Check sheet for the modelled part. Datum: model origin and axes. Units: mm. A direction names the side the tool comes from. Give positions to 0.01 mm unless a question says otherwise; leave off trailing zeros. Write each loop counter-clockwise with the first axis right and the second up, starting at its lowest first coordinate (ties: lowest second). Pieces come first, ordered by that corner, then holes. Notation, with made-up numbers: M -9,71.25 L -1,71.25 A32 ccw -1,103.25 Z; hole C 60,1 d2. An arc over 180 degrees is marked long. Write item = value, one per line. Start each with the question number.
1) Scan lines: L1, parallel to X at y = 25, z = 2; L2, parallel to X at y = 78.5, z = 4; L3, parallel to Y at x = -40, z = -15 (3 decimals). Record each from-to range of solid material in increasing order.
2) Sectioned sample at C-C, the plane y = 97. Record the cut outline in (x, z).
3) Gauge pin test, flat ends, axial feed: pin 1 (11 mm diameter, centred on x = 0, z = -22.225, fed in from +Y) (3 decimals); pin 2 (6 mm diameter, centred on x = -20.5, y = 72, fed in from -Z); pin 3 (5.5 mm diameter, centred on x = 31.81, z = 0, fed in from +Y). Record the tip position at first contact, or that the pin passes through.
4) Sectioned sample at B-B, the plane y = 25.4. Record the cut outline in (x, z).
5) Sectioned sample at A-A, the plane x = -31.75. Count the separate pieces of the cut face and the enclosed holes in it, then the cut area to 3 significant figures.
6) Draft check along X on faces 4 (the face through (10.554, 119.867, 1.612)), 5 (the face through (-1, 3.175, -16)), 6 (the face through (-44.45, 56, -3)). Enter one of: pulls with the +X half, pulls with the -X half, needs draft (parallel to the pull), parting line crosses it, or undercut.
7) Set-up check for faces 1 (the face through (44.45, 56, -3)), 2 (the face through (0.6, 119.062, 0.1)), 3 (the face through (21.4, 119.87, 3.23)): record each of +Z, -Z, +X, -X, +Y, -Y from which the full face is reachable in a straight line by a thin tool's end or side.
from build123d import *

# Parameters (mm, degrees)
SKETCH1_W               = 88.9
SKETCH1_H               = 12.7
BOSS_EXTRUDE1_DEPTH     = 76.2
SKETCH2_R               = 3.4925
BOSS_EXTRUDE4_DEPTH     = 3.175
BOSS_EXTRUDE5_DEPTH     = 12.7
CUT_EXTRUDE1_REACH      = 134.44
SKETCH4_R               = 3.4925
CUT_EXTRUDE2_DEPTH      = 133.439750453
CUT_EXTRUDE2_DEPTH_BACK = 133.439750453
SKETCH5_R               = 3.4925


with BuildPart() as part:
    # Sketch1 → Boss-Extrude1 (new body)
    with BuildSketch(Plane(origin=(0, 0, 0), x_dir=(1, 0, 0), z_dir=(0, 1, 0))):
        Rectangle(SKETCH1_W, SKETCH1_H)
    extrude(amount=BOSS_EXTRUDE1_DEPTH)

    # Sketch2 → Boss-Extrude4 (add)
    with BuildSketch(Plane(origin=(0, 0, 0), x_dir=(1, 0, 0), z_dir=(0, 1, 0))):
        Polygon((-44.45, 22.225), (-44.45, 6.35), (44.45, 6.35), (44.45, 31.75), (-44.45, 31.75), align=None)
        with Locations(Location((-25.4, 22.225, 0), (0, 0, 270))):
            Circle(SKETCH2_R, mode=Mode.SUBTRACT)
        with Locations(Location((0, 22.225, 0), (0, 0, 270))):
            Circle(SKETCH2_R, mode=Mode.SUBTRACT)
        with Locations(Location((25.4, 22.225, 0), (0, 0, 270))):
            Circle(SKETCH2_R, mode=Mode.SUBTRACT)
    extrude(amount=BOSS_EXTRUDE4_DEPTH)

    # Sketch3 → Boss-Extrude5 (add)
    with BuildSketch(Plane.XY.offset(6.35)):
        Polygon((-44.45, 76.2), (-44.45, 120.65), (44.45, 120.65), (44.45, 76.2), (42.8625, 76.2), (42.8625, 119.0625), (-42.8625, 119.0625), (-42.8625, 76.2), align=None)
    extrude(amount=-BOSS_EXTRUDE5_DEPTH)

    # Sketch4 → Cut-Extrude1 (cut, up to next)
    with BuildSketch(Plane(origin=(0, 120.65, 0), x_dir=(1, 0, 0), z_dir=(0, 1, 0)), mode=Mode.PRIVATE) as cut_extrude1_sk1:
        with Locations(Location((-31.75, 0, 0), (0, 0, 270))):
            Circle(SKETCH4_R)
    cut_extrude1_tool1 = extrude(cut_extrude1_sk1.sketch, amount=-CUT_EXTRUDE1_REACH, mode=Mode.PRIVATE) & part.part
    # Sketch4 → Cut-Extrude1 (cut, up to next)
    with BuildSketch(Plane(origin=(0, 120.65, 0), x_dir=(1, 0, 0), z_dir=(0, 1, 0)), mode=Mode.PRIVATE) as cut_extrude1_sk2:
        with Locations(Location((-22.6695, 0, 0), (0, 0, 270))):
            Circle(SKETCH4_R)
    cut_extrude1_tool2 = extrude(cut_extrude1_sk2.sketch, amount=-CUT_EXTRUDE1_REACH, mode=Mode.PRIVATE) & part.part
    # Sketch4 → Cut-Extrude1 (cut, up to next)
    with BuildSketch(Plane(origin=(0, 120.65, 0), x_dir=(1, 0, 0), z_dir=(0, 1, 0)), mode=Mode.PRIVATE) as cut_extrude1_sk3:
        with Locations(Location((-13.589, 0, 0), (0, 0, 270))):
            Circle(SKETCH4_R)
    cut_extrude1_tool3 = extrude(cut_extrude1_sk3.sketch, amount=-CUT_EXTRUDE1_REACH, mode=Mode.PRIVATE) & part.part
    # Sketch4 → Cut-Extrude1 (cut, up to next)
    with BuildSketch(Plane(origin=(0, 120.65, 0), x_dir=(1, 0, 0), z_dir=(0, 1, 0)), mode=Mode.PRIVATE) as cut_extrude1_sk4:
        with Locations(Location((-4.5085, 0, 0), (0, 0, 270))):
            Circle(SKETCH4_R)
    cut_extrude1_tool4 = extrude(cut_extrude1_sk4.sketch, amount=-CUT_EXTRUDE1_REACH, mode=Mode.PRIVATE) & part.part
    # Sketch4 → Cut-Extrude1 (cut, up to next)
    with BuildSketch(Plane(origin=(0, 120.65, 0), x_dir=(1, 0, 0), z_dir=(0, 1, 0)), mode=Mode.PRIVATE) as cut_extrude1_sk5:
        with Locations(Location((4.572, 0, 0), (0, 0, 270))):
            Circle(SKETCH4_R)
    cut_extrude1_tool5 = extrude(cut_extrude1_sk5.sketch, amount=-CUT_EXTRUDE1_REACH, mode=Mode.PRIVATE) & part.part
    # Sketch4 → Cut-Extrude1 (cut, up to next)
    with BuildSketch(Plane(origin=(0, 120.65, 0), x_dir=(1, 0, 0), z_dir=(0, 1, 0)), mode=Mode.PRIVATE) as cut_extrude1_sk6:
        with Locations(Location((13.6525, 0, 0), (0, 0, 270))):
            Circle(SKETCH4_R)
    cut_extrude1_tool6 = extrude(cut_extrude1_sk6.sketch, amount=-CUT_EXTRUDE1_REACH, mode=Mode.PRIVATE) & part.part
    # Sketch4 → Cut-Extrude1 (cut, up to next)
    with BuildSketch(Plane(origin=(0, 120.65, 0), x_dir=(1, 0, 0), z_dir=(0, 1, 0)), mode=Mode.PRIVATE) as cut_extrude1_sk7:
        with Locations(Location((22.733, 0, 0), (0, 0, 270))):
            Circle(SKETCH4_R)
    cut_extrude1_tool7 = extrude(cut_extrude1_sk7.sketch, amount=-CUT_EXTRUDE1_REACH, mode=Mode.PRIVATE) & part.part
    # Sketch4 → Cut-Extrude1 (cut, up to next)
    with BuildSketch(Plane(origin=(0, 120.65, 0), x_dir=(1, 0, 0), z_dir=(0, 1, 0)), mode=Mode.PRIVATE) as cut_extrude1_sk8:
        with Locations(Location((31.8135, 0, 0), (0, 0, 270))):
            Circle(SKETCH4_R)
    cut_extrude1_tool8 = extrude(cut_extrude1_sk8.sketch, amount=-CUT_EXTRUDE1_REACH, mode=Mode.PRIVATE) & part.part
    add(cut_extrude1_tool1.solids().sort_by_distance((-31.75, 120.65, 0))[0], mode=Mode.SUBTRACT)
    add(cut_extrude1_tool2.solids().sort_by_distance((-22.6695, 120.65, 0))[0], mode=Mode.SUBTRACT)
    add(cut_extrude1_tool3.solids().sort_by_distance((-13.589, 120.65, 0))[0], mode=Mode.SUBTRACT)
    add(cut_extrude1_tool4.solids().sort_by_distance((-4.5085, 120.65, 0))[0], mode=Mode.SUBTRACT)
    add(cut_extrude1_tool5.solids().sort_by_distance((4.572, 120.65, 0))[0], mode=Mode.SUBTRACT)
    add(cut_extrude1_tool6.solids().sort_by_distance((13.6525, 120.65, 0))[0], mode=Mode.SUBTRACT)
    add(cut_extrude1_tool7.solids().sort_by_distance((22.733, 120.65, 0))[0], mode=Mode.SUBTRACT)
    add(cut_extrude1_tool8.solids().sort_by_distance((31.8135, 120.65, 0))[0], mode=Mode.SUBTRACT)

    # Sketch5 → Cut-Extrude2 (cut, two sides: drawn at the far end of the back side and taken through both)
    with BuildSketch(Plane.XY.offset(-CUT_EXTRUDE2_DEPTH_BACK)):
        with Locations((-19.05, 25.4)):
            Circle(SKETCH5_R)
        with Locations((19.05, 25.4)):
            Circle(SKETCH5_R)
    extrude(amount=CUT_EXTRUDE2_DEPTH + CUT_EXTRUDE2_DEPTH_BACK, mode=Mode.SUBTRACT)


solid = part.part
Data:
q1.L1 = -44.45 to -22.52, -15.58 to 15.58, 22.52 to 44.45
q1.L2 = -44.45 to -42.86, 42.86 to 44.45
q1.L3 = 0 to 3.175
q2.outline = M -44.45,-6.35 L -42.86,-6.35 L -42.86,6.35 L -44.45,6.35 Z; M 42.86,-6.35 L 44.45,-6.35 L 44.45,6.35 L 42.86,6.35 Z
q3.pin_1 = 3.175
q3.pin_2 = -6.35
q3.pin_3 = 76.2
q4.outline = M -44.45,-6.35 L -22.54,-6.35 L -22.54,6.35 L -44.45,6.35 Z; M -15.56,-6.35 L 15.56,-6.35 L 15.56,6.35 L -15.56,6.35 Z; M 22.54,-6.35 L 44.45,-6.35 L 44.45,6.35 L 22.54,6.35 Z
q5.separate_pieces = 3
q5.enclosed_holes = 0
q5.area = 1,060 mm2
q6.face_4 = undercut
q6.face_5 = needs draft
q6.face_6 = pulls with the -X half
q7.face_1 = +Z, -Z, +X, +Y, -Y
q7.face_2 = +Z, -Z
q7.face_3 = +Y
